Design review of the part built by this model. Coordinates are the model's own, in mm. A direction names the side the tool comes from. Coordinates: 2 decimals unless noted, no trailing zeros. Loops run counter-clockwise (first coordinate to the right, second up) from the corner with the lowest first, then second, coordinate; pieces in that order, holes last.
Q1. Draft analysis for pull direction X (two halves, no side actions). For faces 3 (the face through (0, 0, 1.5)), 4 (the face through (-0.434, -1.952, 0.493)), 5 (the face through (-1, -1, 4.5)), 6 (the face through (0, -1, 3)), state which applies: released by +X, released by -X, zero draft, split by the parting line, or undercut.
Q2. For P1, Ø0.5, axis at x = 0, y = 2, coming from the -Z side, flat-tipped, find the tip position at first contact; note if it passes through.
Q3. Machinability: for faces 1 (the face through (1, -1, 0)), 2 (the face through (0, 0, -4.3)), which of the approach directions +Z, -Z, +X, -X, +Y, -Y give a long, thin tool a straight path to every point of the face, cutting with its end or side? Answer none if there is none.
Q4. Add section B-B on y = -1.1. Give the boundary of the cut face in (x, z), and give its area (3 significant figures).
Q5. Add section A-A on z = -3.5. Give the boundary of the cut face in (x, y).
Q6. Wall thickness on probe 1 along Z at (x, y) = (0.85, -0.65); probe 2 along X at (y, z) = (0.9, 2.5); probe 3 along Y at (x, z) = (0.75, 2.5): over which ranges is each line inside the solid? List them lowest first.
```python
from build123d import *

# Parameters (mm, degrees)
SKETCH_1_R          = 1
EXTRUDE_1_DEPTH     = 4.3
SKETCH_2_R          = 2
EXTRUDE_2_DEPTH     = 1
EXTRUDE_3_DEPTH     = 3.5
SKETCH_4_R          = 1
CUT_EXTRUDE_1_DEPTH = 3


with BuildPart() as part:
    # 草图1 → 凸台-拉伸1 (new body)
    with BuildSketch(Plane.XY):
        Circle(SKETCH_1_R)
    extrude(amount=-EXTRUDE_1_DEPTH)

    # 草图2 → 凸台-拉伸2 (add)
    with BuildSketch(Plane.XY):
        Circle(SKETCH_2_R)
    extrude(amount=EXTRUDE_2_DEPTH)

    # 草图3 → 凸台-拉伸3 (add)
    with BuildSketch(Plane.XY.offset(1)):
        Polygon((2.359708326, -0.825697655), (1.801937736, -0.867767478), (2.116810498, -1.330080191), (1.563662965, -1.246979604), (1.767766953, -1.767766953), (1.246979604, -1.563662965), (1.330080191, -2.116810498), (0.867767478, -1.801937736), (0.825697655, -2.359708326), (0.445041868, -1.949855824), (0.27991119, -2.484280525), (0, -2), (-0.27991119, -2.484280525), (-0.445041868, -1.949855824), (-0.825697655, -2.359708326), (-0.867767478, -1.801937736), (-1.330080191, -2.116810498), (-1.246979604, -1.563662965), (-1.767766953, -1.767766953), (-1.563662965, -1.246979604), (-2.116810498, -1.330080191), (-1.801937736, -0.867767478), (-2.359708326, -0.825697655), (-1.949855824, -0.445041868), (-2.484280525, -0.27991119), (-2, 0), (-2.484280525, 0.27991119), (-1.949855824, 0.445041868), (-2.359708326, 0.825697655), (-1.801937736, 0.867767478), (-2.116810498, 1.330080191), (-1.563662965, 1.246979604), (-1.767766953, 1.767766953), (-1.246979604, 1.563662965), (-1.330080191, 2.116810498), (-0.867767478, 1.801937736), (-0.825697655, 2.359708326), (-0.445041868, 1.949855824), (-0.27991119, 2.484280525), (0, 2), (0.27991119, 2.484280525), (0.445041868, 1.949855824), (0.825697655, 2.359708326), (0.867767478, 1.801937736), (1.330080191, 2.116810498), (1.246979604, 1.563662965), (1.767766953, 1.767766953), (1.563662965, 1.246979604), (2.116810498, 1.330080191), (1.801937736, 0.867767478), (2.359708326, 0.825697655), (1.949855824, 0.445041868), (2.484280525, 0.27991119), (2, 0), (2.484280525, -0.27991119), (1.949855824, -0.445041868), align=None)
    extrude(amount=EXTRUDE_3_DEPTH)

    # 草图4 → 切除-拉伸1 (cut)
    with BuildSketch(Plane.XY.offset(4.5)):
        Circle(SKETCH_4_R)
    extrude(amount=-CUT_EXTRUDE_1_DEPTH, mode=Mode.SUBTRACT)


solid = part.part
```
Entries:
1. face 3: undercut
1. face 4: split by the parting line
1. face 5: zero draft
1. face 6: undercut
2. P1: stops at z = 0
3. face 1: -Z
3. face 2: -Z, +X, -X, +Y, -Y
4. outline: (-1.96, 1) - (-1.67, 1) - (-1.67, 0) - (1.67, 0) - (1.67, 1) - (1.96, 1) - (1.96, 4.5) - (-1.96, 4.5) - close
4. area: 17.1 mm2
5. outline: circle Ø2 at (0, 0)
6. probe 1: z = 0 to 4.5
6. probe 2: x = -1.82 to -0.44, 0.44 to 1.82
6. probe 3: y = -2.28 to -0.66, 0.66 to 2.28
